Print and shaded views of the part. All mm, measured from the part's lowest x, y and z. Coordinates: 2 decimals unless noted, no trailing zeros. Order: outer loops, then holes, each group sorted by start corner. A loop starts at its lowest first (then second) coordinate and runs counter-clockwise, first axis right, second up. Notation, with made-up numbers: M 41.25,50.5 L 94.25,50.5 A17 cw 94.25,63.5 Z; hole C 8,40 d2. An arc over 180 degrees is marked long. Use a Markdown table: item, result. Add a question column.
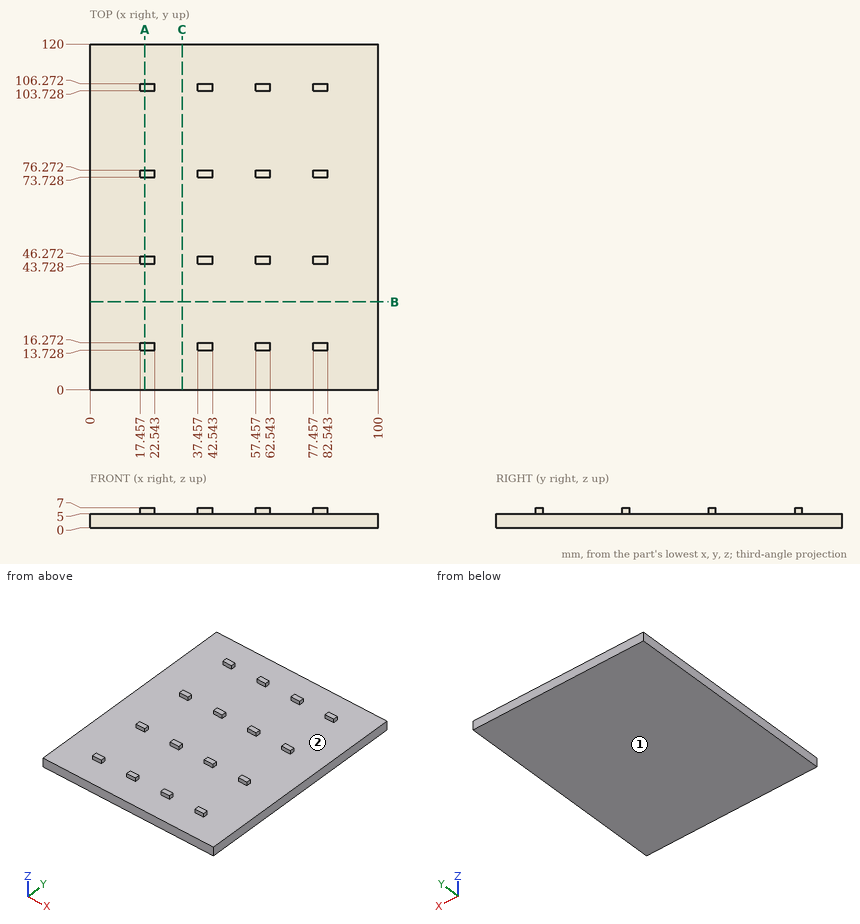
(1) Mould opens along Y. For the marked faces 1 and 2 say: released by +Y, released by -Y, zero draft, split by the parting line, or undercut.
(2) Drop flat-ended pins along their axis: P1, Ø1, axis at y = 74.5, z = 6.5, coming from the +X side; P2, Ø1, axis at x = 40, z = 6.5, coming from the -Y side; P3, Ø1, axis at x = 60, z = 6, coming from the +Y side; P4, Ø2, axis at x = 50.5, y = 25.5, coming from the -Z side. Give the stop position or say it passes through.
(3) Slice it at A-A on x = 19. Give the cut face in (y, z).
(4) Slice it at C-C on x = 32. Give the cut face in (y, z).
(5) Drill centre line: line 1 along Z through (x, y) = (46.5, 59.5). Where is it in solid material? Low to high. Write a range as from..to.
(6) Slice it at B-B on y = 30.5. Give the cut face in (x, z).
Solutions:
| question | item | result |
|---|---|---|
| 1 | face 1 | zero draft |
| 1 | face 2 | undercut |
| 2 | P1 | x = 82.54 |
| 2 | P2 | y = 13.73 |
| 2 | P3 | y = 106.27 |
| 2 | P4 | z = 0 |
| 3 | outline | M 0,0 L 120,0 L 120,5 L 106.27,5 L 106.27,7 L 103.73,7 L 103.73,5 L 76.27,5 L 76.27,7 L 73.73,7 L 73.73,5 L 46.27,5 L 46.27,7 L 43.73,7 L 43.73,5 L 16.27,5 L 16.27,7 L 13.73,7 L 13.73,5 L 0,5 Z |
| 4 | outline | M 0,0 L 120,0 L 120,5 L 0,5 Z |
| 5 | line 1 | 0..5 |
| 6 | outline | M 0,0 L 100,0 L 100,5 L 0,5 Z |
